Geometry: see drawing. Coordinates: mm, zero at the bounding-box minimum. A direction names the side the tool comes from. Coordinates: 2 decimals unless noted, no trailing zeros. Loops run counter-clockwise (first coordinate to the right, second up) from the corner with the lowest first, then second, coordinate; pieces in that order, holes last. Notation, with made-up numbers: (12.5, 51) - (64.5, 51) arc R31 cw to (64.5, 86) - close; hole circle Ø7 at (81.5, 60). An arc over 180 degrees is marked (long way). Answer in a Markdown table with one row per item.
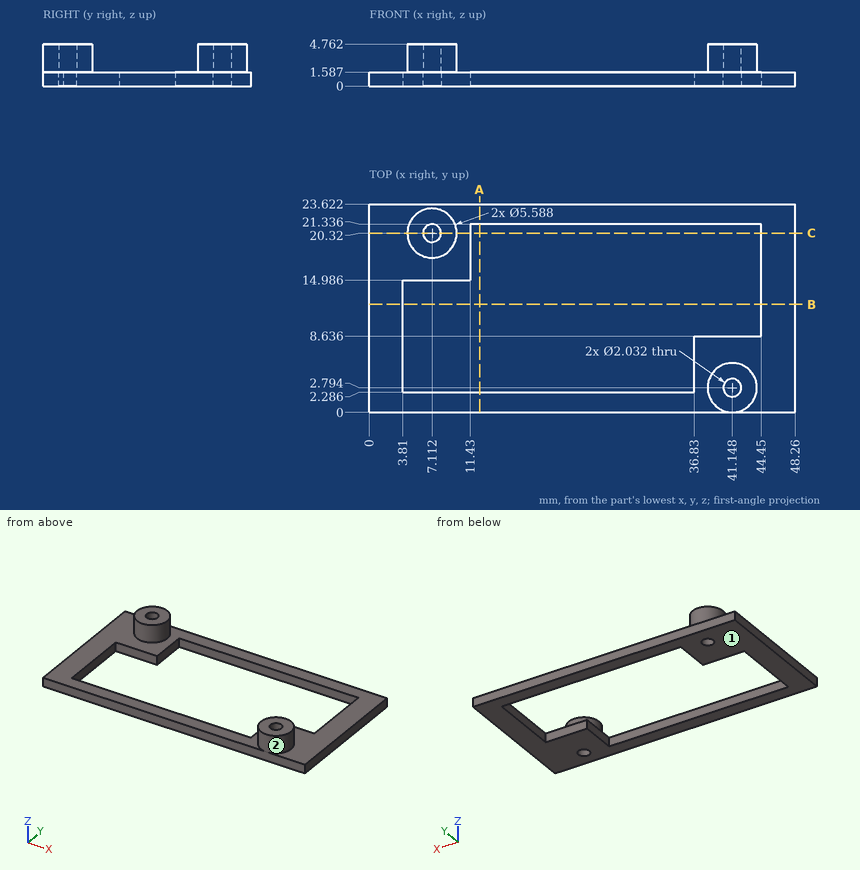
(1) Cut plane A-A on x = 12.5. Output: boundary loops of the cut face in (y, z) (1 decimal).
Verdict:
| item | result |
|---|---|
| outline | (0, 0) - (2.3, 0) - (2.3, 1.6) - (0, 1.6) - close; (21.3, 0) - (23.6, 0) - (23.6, 1.6) - (21.3, 1.6) - close |
(2) First-contact query: pin 1 Ø8 at (x, y) = (7.5, 4) entering from +Z. Flat tip, straight axial feed; report the tip coordinate or a pass-through.
Verdict:
| item | result |
|---|---|
| pin 1 | stops at z = 1.59 |
(3) Cut plane B-B on y = 12.25. Output: boundary loops of the cut face in (x, z).
Verdict:
| item | result |
|---|---|
| outline | (0, 0) - (3.81, 0) - (3.81, 1.59) - (0, 1.59) - close; (44.45, 0) - (48.26, 0) - (48.26, 1.59) - (44.45, 1.59) - close |
(4) Ray query, probe 1 along Y at (x, z) = (41, 1.45) (1 decimal); probe 2 along Y at (x, z) = (15.5, 1) (1 decimal); probe 3 along X at (y, z) = (4.25, 0.7). Return the intervals inside material, ascending.
Verdict:
| item | result |
|---|---|
| probe 1 | y = 0 to 1.8, 3.8 to 8.6, 21.3 to 23.6 |
| probe 2 | y = 0 to 2.3, 21.3 to 23.6 |
| probe 3 | x = 0 to 3.81, 36.83 to 48.26 |
(5) Cut plane C-C on y = 20.32. State how many separate pieces and enclosed holes the cut face has.
Verdict:
| item | result |
|---|---|
| separate pieces | 3 |
| enclosed holes | 0 |
(6) Access query for the marked faces 1 and 2. Directions: +Z, -Z, +X, -X, +Y, -Y. A direction counts if a zero-diameter tool reaches every point of the face in a straight line with its end or side. Return the directions, or none.
Verdict:
| item | result |
|---|---|
| face 1 | -Z, +X, -X, +Y, -Y |
| face 2 | +Z |
